```python
from build123d import *

# Parameters (mm, degrees)
SKETCH_1_R      = 3
SKETCH_1_R_2    = 1.5
EXTRUDE_1_DEPTH = 1.25
EXTRUDE_START   = -0.6
SKETCH_2_R      = 3.6
SKETCH_2_R_2    = 3
EXTRUDE_2_DEPTH = 0.6
CHAMFER_1_SIZE  = 0.1


with BuildPart() as part:
    # 草图1 → 凸台-拉伸1 (new, symmetric)
    with BuildSketch(Plane.XY):
        Circle(SKETCH_1_R)
        Circle(SKETCH_1_R_2, mode=Mode.SUBTRACT)
    extrude(amount=EXTRUDE_1_DEPTH, both=True)

    # 草图2 → 凸台-拉伸2 (add)
    with BuildSketch(Plane(origin=(0, 0, -1.25), x_dir=(-1, 0, 0), z_dir=(0, 0, -1)).offset(EXTRUDE_START)):
        Circle(SKETCH_2_R)
        Circle(SKETCH_2_R_2, mode=Mode.SUBTRACT)
    extrude(amount=EXTRUDE_2_DEPTH)

    # 倒角1
    chamfer_1_edges = [part.edges().sort_by_distance(p)[0] for p in [
        (3.6, 0, -0.65),
        (3.6, 0, -1.25),
        (-3, 0, 1.25),
        (-1.5, 0, -1.25),
        (-1.5, 0, 1.25),
    ]]
    chamfer(chamfer_1_edges, length=CHAMFER_1_SIZE)


solid = part.part
```
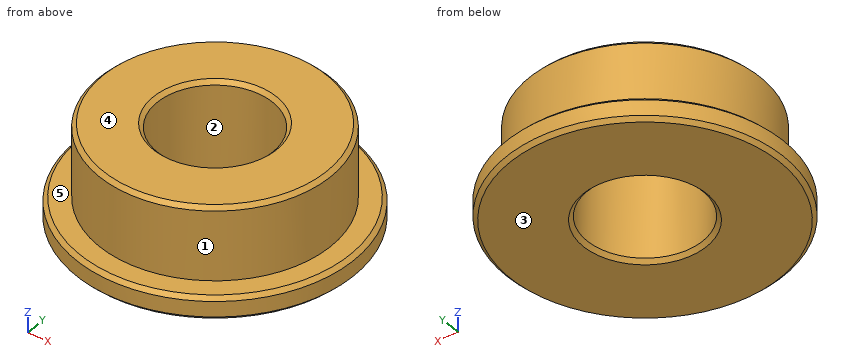
Model file for the job. Use its own axes, mm. Face numbers are marked on the shaded views. A direction names the side the tool comes from. Coordinates: 2 decimals unless noted, no trailing zeros. Order: outer loops, then holes, each group sorted by start corner. A loop starts at its lowest first (then second) coordinate and runs counter-clockwise, first axis right, second up. Notation, with made-up numbers: (23, -12.75) - (60, -12.75) arc R25 ccw to (60, 24.25) - close; hole circle Ø11 at (4.25, 66). An arc over 180 degrees is marked (long way). Return JSON: item names as keys, results as strings. Group by question number.
1) Mould opens along Y. For the marked faces 1, 2 and 3 say: released by +Y, released by -Y, zero draft, split by the parting line, or undercut.
2) Saw through at D-D, the plane z = -0.95. Write the cut outline in (x, y), plus the area to 3 significant figures.
3) Saw through at C-C, the plane z = 0.3. Write the cut outline in (x, y).
4) Probe line 1 (Y direction, x = 0, z = 0.25); line 2 (Z direction, x = 3, y = -0.75); line 3 (X direction, y = -0.75, z = -0.8). List the from-to ranges inside material, lowest first. Write a range as from..to.
5) Tool access for the marked faces 4 and 5: list every direction of +Z, -Z, +X, -X, +Y, -Y with a clear straight run to the whole face (end or side of a thin tool).
6) Saw through at A-A, the plane x = 0. Write the cut outline in (y, z), plus the area to 3 significant figures.
7) Flat gauge pin, fed straight in: P1, Ø1.5, axis at x = -1, z = 1, coming from the -Y side. Where does the tip first touch, or does it go through?
Values found:
{
 "1": {"face 1": "split by the parting line", "face 2": "undercut", "face 3": "zero draft"},
 "2": {"outline": "circle Ø7.2 at (0, 0); hole circle Ø3 at (0, 0)", "area": "33.6 mm²"},
 "3": {"outline": "circle Ø6 at (0, 0); hole circle Ø3 at (0, 0)"},
 "4": {"line 1": "y = -3..-1.5, 1.5..3", "line 2": "z = -1.25..-0.65", "line 3": "x = -3.52..-1.3, 1.3..3.52"},
 "5": {"face 4": "+Z, +X, -X, +Y, -Y", "face 5": "+Z"},
 "6": {"outline": "(-3.6, -1.15) - (-3.5, -1.25) - (-1.6, -1.25) - (-1.5, -1.15) - (-1.5, 1.15) - (-1.6, 1.25) - (-2.9, 1.25) - (-3, 1.15) - (-3, -0.65) - (-3.5, -0.65) - (-3.6, -0.75) - close; (1.5, -1.15) - (1.6, -1.25) - (3.5, -1.25) - (3.6, -1.15) - (3.6, -0.75) - (3.5, -0.65) - (3, -0.65) - (3, 1.15) - (2.9, 1.25) - (1.6, 1.25) - (1.5, 1.15) - close", "area": "8.17 mm²"},
 "7": {"P1": "stops at y = -2.99"}
}
